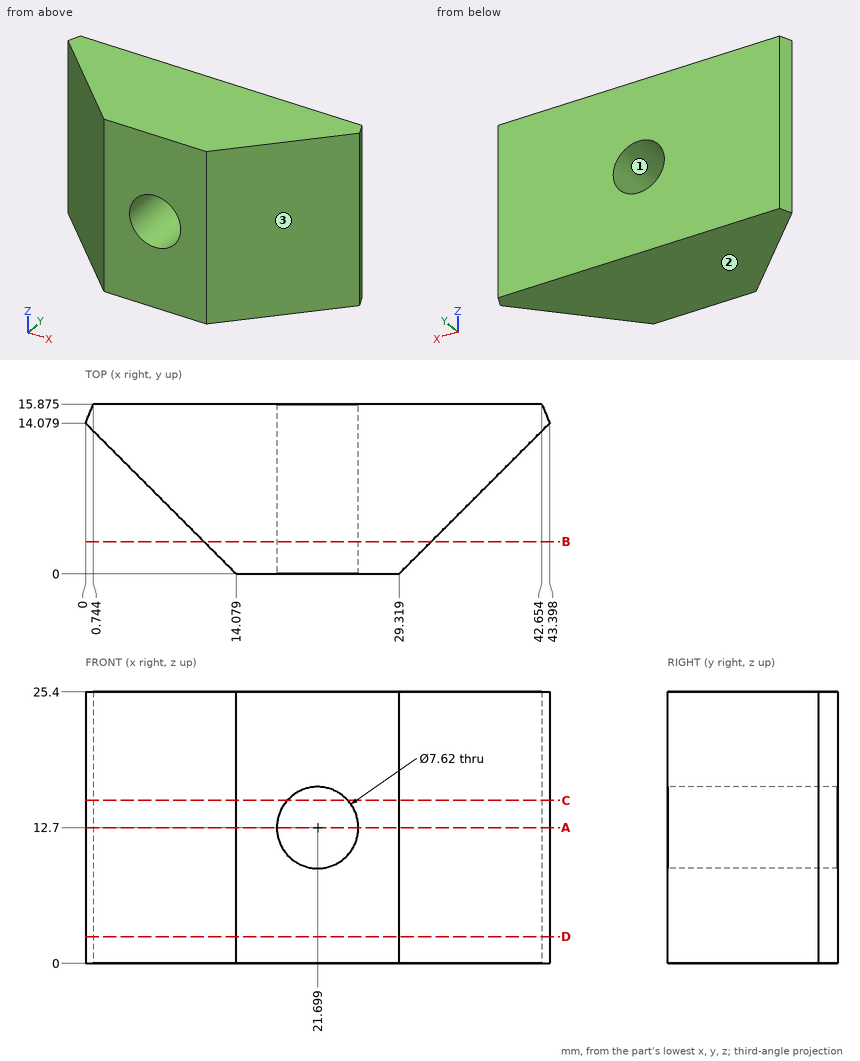
Verification items for this drawing (mm, ordinates from the low corner). Coordinates: 2 decimals unless noted, no trailing zeros. Order: outer loops, then holes, each group sorted by start corner. A loop starts at its lowest first (then second) coordinate and runs counter-clockwise, first axis right, second up.
Q1. Sectioned sample at A-A on z = 12.7. Record the cut outline in (x, y) (3 decimals), and give its area (3 significant figures).
Reply:
outline: (0, 14.079) - (14.079, 0) - (17.889, 0) - (17.889, 15.875) - (0.744, 15.875) - close; (25.509, 0) - (29.319, 0) - (43.398, 14.079) - (42.654, 15.875) - (25.509, 15.875) - close
area: 368 mm2
Q2. Depth check by flat-ended pin: pin 1 Ø2 at (y, z) = (11, 19.5) entering from +X; pin 2 Ø9 at (x, z) = (21.7, 12.7) entering from +Y (3 decimals); pin 3 Ø4 at (x, z) = (7, 20) entering from -Y; pin 4 Ø3 at (y, z) = (7, 17.5) entering from -X. Enter the tip coordinate at first touch or a pass-through.
Reply:
pin 1: stops at x = 41.32
pin 2: stops at y = 15.875
pin 3: stops at y = 5.08
pin 4: stops at x = 5.58
Q3. Sectioned sample at C-C on z = 15.25. Record the cut outline in (x, y) (3 decimals).
Reply:
outline: (0, 14.079) - (14.079, 0) - (18.868, 0) - (18.868, 15.875) - (0.744, 15.875) - close; (24.53, 0) - (29.319, 0) - (43.398, 14.079) - (42.654, 15.875) - (24.53, 15.875) - close
Q4. Thickness scan on probe 1 along Z at (x, y) = (20, 7.75); probe 2 along X at (y, z) = (11, 17.25); probe 3 along X at (y, z) = (6.5, 21). Record the ranges inside material, lowest first.
Reply:
probe 1: z = 0 to 9.29, 16.11 to 25.4
probe 2: x = 3.08 to 40.32
probe 3: x = 7.58 to 35.82
Q5. Sectioned sample at B-B on y = 3. Record the cut outline in (x, z).
Reply:
outline: (11.08, 0) - (32.32, 0) - (32.32, 25.4) - (11.08, 25.4) - close; hole circle Ø7.62 at (21.7, 12.7)
Q6. Draft check along Z on the marked faces 1, 2 and 3. Enter one of: released by +Z, released by -Z, zero draft, split by the parting line, or undercut.
Reply:
face 1: undercut
face 2: released by -Z
face 3: zero draft
Q7. Sectioned sample at D-D on z = 2.5. Record the cut outline in (x, y) (3 decimals).
Reply:
outline: (0, 14.079) - (14.079, 0) - (29.319, 0) - (43.398, 14.079) - (42.654, 15.875) - (0.744, 15.875) - close
